from build123d import *

# Parameters (mm, degrees)
SKETCH1_R           = 26.83
SKETCH1_R_2         = 3.5
SKETCH1_R_3         = 2
BOSS_EXTRUDE1_DEPTH = 2.5
CUT_EXTRUDE2_START  = -10
CUT_EXTRUDE2_DEPTH  = 10
SKETCH2_R           = 1.3
CUT_EXTRUDE3_DEPTH  = 10


with BuildPart() as part:
    # Sketch1 → Boss-Extrude1 (new body)
    with BuildSketch(Plane(origin=(0, 0, 0), x_dir=(1, 0, 0), z_dir=(0, 1, 0))):
        with Locations(Location((0, 0, 0), (0, 0, 270))):
            Circle(SKETCH1_R)
        with Locations(Location((0, 0, 0), (0, 0, 270))):
            Circle(SKETCH1_R_2, mode=Mode.SUBTRACT)
        with Locations(Location((-16.000000001, 16.000000001, 0), (0, 0, 270))):
            Circle(SKETCH1_R_3, mode=Mode.SUBTRACT)
        with Locations(Location((16.000000001, 16.000000001, 0), (0, 0, 270))):
            Circle(SKETCH1_R_3, mode=Mode.SUBTRACT)
        with Locations(Location((16.000000001, -16.000000001, 0), (0, 0, 270))):
            Circle(SKETCH1_R_3, mode=Mode.SUBTRACT)
        with Locations(Location((-16.000000001, -16.000000001, 0), (0, 0, 270))):
            Circle(SKETCH1_R_3, mode=Mode.SUBTRACT)
    extrude(amount=BOSS_EXTRUDE1_DEPTH)

    # Sketch3 → Cut-Extrude2 (cut)
    with BuildSketch(Plane(origin=(0, 2.5, 0), x_dir=(1, 0, 0), z_dir=(0, 1, 0)).offset(CUT_EXTRUDE2_START)):
        with BuildLine():
            Line((-19.833935995, -18.068311569), (-19.833935995, 18.068311569))
            ThreePointArc((-19.833935995, 18.068311569), (-26.83, 0), (-19.833935995, -18.068311569))
        make_face()
        with BuildLine():
            Line((-18.068311569, 19.833935995), (18.068311569, 19.833935995))
            ThreePointArc((18.068311569, 19.833935995), (0, 26.83), (-18.068311569, 19.833935995))
        make_face()
        with BuildLine():
            ThreePointArc((26.83, 0), (25.019926086, 9.687734443), (19.833935995, 18.068311569))
            Line((19.833935995, 18.068311569), (19.833935995, -18.068311569))
            ThreePointArc((19.833935995, -18.068311569), (25.019926086, -9.687734443), (26.83, 0))
        make_face()
        with BuildLine():
            ThreePointArc((-18.068311569, -19.833935995), (0, -26.83), (18.068311569, -19.833935995))
            Line((18.068311569, -19.833935995), (-18.068311569, -19.833935995))
        make_face()
    extrude(amount=CUT_EXTRUDE2_DEPTH, mode=Mode.SUBTRACT)

    # Sketch2 → Cut-Extrude3 (cut)
    with BuildSketch(Plane(origin=(0, 2.5, 0), x_dir=(1, 0, 0), z_dir=(0, 1, 0))):
        with Locations(Location((-5.262430087, 5.262430087, 0), (0, 0, 270))):
            Circle(SKETCH2_R)
        with Locations(Location((5.262430087, -5.262430087, 0), (0, 0, 270))):
            Circle(SKETCH2_R)
    extrude(amount=-CUT_EXTRUDE3_DEPTH, mode=Mode.SUBTRACT)


solid = part.part
Work out the finished part from the listing and answer in its coordinate system (mm). Round coordinates to 2 decimals unless told otherwise and drop trailing zeros. Write each loop counter-clockwise with the first axis right and the second up, starting at its lowest first coordinate (ties: lowest second). Pieces come first, ordered by that corner, then holes. Notation, with made-up numbers: (9, 49) - (64, 49) arc R25 cw to (64, 84) - close; hole circle Ø9 at (-34.5, 80). An arc over 180 degrees is marked (long way). Answer in a Markdown table with one row per item. Add a question column.
1. Given pin 1 (2.5 mm diameter, centred on x = 16, z = -16, fed in from +Y) (3 decimals); pin 2 (5 mm diameter, centred on x = 15, z = -1.5, fed in from -Y), each flat-ended and moving along its own axis, determine where each tip first touches the part or whether it passes through.
2. A cutting plane is placed at A-A, the plane x = 0. Determine the outline of the cut face in (y, z).
3. The mould has two halves that part along Z. Classify faces 1 (the cylindrical face through (-3.417, 1.232, -0.759)), 2 (the flat face through (19.834, 1, 0)), 3 (the cylindrical face through (18.959, 1.232, 18.984)), 4 (the cylindrical face through (-18.959, 1.232, -18.984)): +Z half, -Z half, draft (parallel to the pull), parting line (faces both ways), or undercut.
4. A cutting plane is placed at B-B, the plane z = -16. Determine the outline of the cut face in (x, y).
5. A cutting plane is placed at D-D, the plane z = 0.5. Determine the outline of the cut face in (x, y), and give its area (3 significant figures).
6. Find the intervals of material crossed by line 1 along X through (y, z) = (1.05, -16); line 2 along X through (y, z) = (1.5, 15.5), in increasing order. Write a range as from..to.
7. A cutting plane is placed at C-C, the plane x = -15. Determine the outline of the cut face in (y, z).
Worked out:
| question | item | result |
|---|---|---|
| 1 | pin 1 | through |
| 1 | pin 2 | y = 0 |
| 2 | outline | (0, -19.83) - (2.5, -19.83) - (2.5, -3.5) - (0, -3.5) - close; (0, 3.5) - (2.5, 3.5) - (2.5, 19.83) - (0, 19.83) - close |
| 3 | face 1 | undercut |
| 3 | face 2 | draft |
| 3 | face 3 | +Z half |
| 3 | face 4 | -Z half |
| 4 | outline | (-19.83, 0) - (-18, 0) - (-18, 2.5) - (-19.83, 2.5) - close; (-14, 0) - (14, 0) - (14, 2.5) - (-14, 2.5) - close; (18, 0) - (19.83, 0) - (19.83, 2.5) - (18, 2.5) - close |
| 5 | outline | (-19.83, 0) - (-3.46, 0) - (-3.46, 2.5) - (-19.83, 2.5) - close; (3.46, 0) - (19.83, 0) - (19.83, 2.5) - (3.46, 2.5) - close |
| 5 | area | 81.8 mm^2 |
| 6 | line 1 | -19.83..-18, -14..14, 18..19.83 |
| 6 | line 2 | -19.83..-17.94, -14.06..14.06, 17.94..19.83 |
| 7 | outline | (0, -19.83) - (2.5, -19.83) - (2.5, -17.73) - (0, -17.73) - close; (0, -14.27) - (2.5, -14.27) - (2.5, 14.27) - (0, 14.27) - close; (0, 17.73) - (2.5, 17.73) - (2.5, 19.83) - (0, 19.83) - close |
